The model under review builds one solid part; all positions refer to its coordinate system, in mm. A direction names the side the tool comes from. Coordinates: 2 decimals unless noted, no trailing zeros. Order: outer loops, then holes, each group sorted by start corner. A loop starts at its lowest first (then second) coordinate and runs counter-clockwise, first axis right, second up.
from build123d import *

# Parameters (mm, degrees)
SKETCH_1_W          = 22.9
SKETCH_1_H          = 21
EXTRUDE_1_DEPTH     = 2
SKETCH_2_W          = 4.5
SKETCH_2_H          = 6
EXTRUDE_2_DEPTH     = 14.4
FILLET_1_R          = 1
SKETCH_3_R          = 4
CUT_EXTRUDE_1_DEPTH = 14.4
SKETCH_5_R          = 0.95
CUT_EXTRUDE_2_DEPTH = 14.4
SKETCH_1_2_W        = 22.9
SKETCH_1_2_H        = 21
EXTRUDE_3_DEPTH     = 2
SKETCH_6_R          = 4
CUT_EXTRUDE_3_DEPTH = 1
SKETCH_7_R          = 1.75
CUT_EXTRUDE_4_DEPTH = 1
FILLET_2_R          = 1
SKETCH_9_W          = 22.900603658
SKETCH_9_H          = 0.5
CUT_EXTRUDE_5_DEPTH = 4
FILLET_4_R          = 1
FILLET_5_DEPTH      = 14.4


with BuildPart() as part:
    # 草图1 → 凸台-拉伸1 (new body)
    with BuildSketch(Plane(origin=(0, 0, 0), x_dir=(1, 0, 0), z_dir=(0, 1, 0))):
        Rectangle(SKETCH_1_W, SKETCH_1_H)
    extrude(amount=EXTRUDE_1_DEPTH)

    # 草图2 → 凸台-拉伸2 (add)
    with BuildSketch(Plane(origin=(0, 0, 0), x_dir=(1, 0, 0), z_dir=(0, 1, 0))):
        with Locations((-13.7, -1.1)):
            Rectangle(SKETCH_2_W, SKETCH_2_H)
        with Locations((13.7, -1.1)):
            Rectangle(SKETCH_2_W, SKETCH_2_H)
    extrude(amount=EXTRUDE_2_DEPTH)

    # 圆角1
    fillet_1_edges = [part.edges().sort_by_distance(p)[0] for p in [
        (-11.45, 8.2, 4.1),
        (11.45, 8.2, 4.1),
    ]]
    fillet(fillet_1_edges, radius=FILLET_1_R)

    # 草图3 → 切除-拉伸1 (cut)
    with BuildSketch(Plane(origin=(0, 2, 0), x_dir=(1, 0, 0), z_dir=(0, 1, 0))):
        with Locations(Location((-0.63, -1.66, 0), (0, 0, 270))):
            Circle(SKETCH_3_R)
    extrude(amount=-CUT_EXTRUDE_1_DEPTH, mode=Mode.SUBTRACT)

    # 草图5 → 切除-拉伸2 (cut)
    with BuildSketch(Plane.XY.offset(4.1)):
        with Locations((-13.85, 8.2)):
            Circle(SKETCH_5_R)
        with Locations((13.85, 8.2)):
            Circle(SKETCH_5_R)
    extrude(amount=-CUT_EXTRUDE_2_DEPTH, mode=Mode.SUBTRACT)

    # 草图1<2> → 凸台-拉伸3 (add)
    with BuildSketch(Plane(origin=(0, 0, 0), x_dir=(1, 0, 0), z_dir=(0, 1, 0))):
        Rectangle(SKETCH_1_2_W, SKETCH_1_2_H)
    extrude(amount=-EXTRUDE_3_DEPTH)

    # 草图6 → 切除-拉伸3 (cut)
    with BuildSketch(Plane(origin=(0, 0, 0), x_dir=(1, 0, 0), z_dir=(0, 1, 0))):
        with Locations(Location((-0.63, -1.66, 0), (0, 0, 270))):
            Circle(SKETCH_6_R)
    extrude(amount=-CUT_EXTRUDE_3_DEPTH, mode=Mode.SUBTRACT)

    # 草图7 → 切除-拉伸4 (cut)
    with BuildSketch(Plane(origin=(0, -1, 0), x_dir=(1, 0, 0), z_dir=(0, 1, 0))):
        with Locations(Location((-0.63, -1.66, 0), (0, 0, 270))):
            Circle(SKETCH_7_R)
    extrude(amount=-CUT_EXTRUDE_4_DEPTH, mode=Mode.SUBTRACT)

    # 圆角2
    fillet_2_edges = [part.edges().sort_by_distance(p)[0] for p in [
        (11.45, 0, -10.5),
        (-11.45, 0, -10.5),
    ]]
    fillet(fillet_2_edges, radius=FILLET_2_R)

    # 草图9 → 切除-拉伸5 (cut)
    with BuildSketch(Plane(origin=(0, 2, 0), x_dir=(1, 0, 0), z_dir=(0, 1, 0))):
        with Locations((-0.000301829, -10.25)):
            Rectangle(SKETCH_9_W, SKETCH_9_H)
    extrude(amount=-CUT_EXTRUDE_5_DEPTH, mode=Mode.SUBTRACT)

    # 圆角4
    fillet_4_edges = [part.edges().sort_by_distance(p)[0] for p in [
        (-11.45, 0, 10),
        (11.45, 0, 10),
    ]]
    fillet(fillet_4_edges, radius=FILLET_4_R)

    # 圆角5: read off the stored shape, not the designer's step
    # 圆角5 outline → 圆角5 (cut)
    with BuildSketch(Plane(origin=(0, 0, 0), x_dir=(1, 0, 0), z_dir=(0, 1, 0))):
        with BuildLine():
            ThreePointArc((11.45, 1.9), (14.69341649, -0.235240405), (15.95, -3.909475019))
            Line((15.95, -3.909475019), (15.95, 1.9))
            Line((15.95, 1.9), (11.45, 1.9))
        make_face()
        with BuildLine():
            ThreePointArc((-15.95, -3.909475019), (-14.69341649, -0.235240405), (-11.45, 1.9))
            Line((-11.45, 1.9), (-15.95, 1.9))
            Line((-15.95, 1.9), (-15.95, -3.909475019))
        make_face()
    extrude(amount=FILLET_5_DEPTH, mode=Mode.SUBTRACT)


solid = part.part
(1) Consider section C-C (x = -0.63). Give the boundary of the cut face in (y, z).
(2) Consider section A-A (y = 12.75). Give the boundary of the cut face in (x, z), then the cut area to 3 significant figures.
(3) Wall thickness on line 1 (X direction, y = 8.2, z = 2); line 2 (Y direction, x = -13.85, z = 1.3); line 3 (X direction, y = -0.15, z = 1.66): over which ranges is each line inside the solid? List them lowest first.
(4) Tool access review of faces 1 (the face through (-11.45, 8, 1)), 2 (the face through (13, 0, 2)), 3 (the face through (-1.5, -1, 3.4)), 4 (the face through (14, 7, 4.1)): name each direction out of +Z, -Z, +X, -X, +Y, -Y from which nothing blocks a thin tool from reaching the whole face with its end or side.
(5) The part is to be moulded in two halves that separate along Z. For faces 5 (the face through (0, 2, -3)), 6 (the face through (-0.55, -1.49, -0.09)), 7 (the face through (11.735, 8.287, 3.799)), say which applies: +Z half, -Z half, draft (parallel to the pull), parting line (faces both ways), or undercut.
(6) Consider section D-D (y = 1.5). Give the boundary of the cut face in (x, z).
(7) Consider section B-B (z = 1.66). Give the boundary of the cut face in (x, y), then the cut area to 3 significant figures.
(8) Insertion check: pin 1 Ø3.5 at (x, y) = (12.5, 4) entering from +Z; pin 2 Ø8 at (y, z) = (7.5, 0.5) entering from +X; pin 3 Ø1.5 at (x, y) = (-9.5, 10.5) entering from -Z; pin 4 Ø3.5 at (x, z) = (14.5, 2) entering from -Y. Each pin has a flat end and moves straight along its axis. Give the tip position at first contact, or say it passes through.
Findings:
1. outline: (-2, -10.5) - (2, -10.5) - (2, -2.34) - (-1, -2.34) - (-1, -0.09) - (-2, -0.09) - close; (-2, 3.41) - (-1, 3.41) - (-1, 5.66) - (2, 5.66) - (2, 10) - (-2, 10) - close
2. outline: (-15.95, 3.91) arc R6 ccw to (-11.45, -1.9) - (-11.45, 3.1) arc R1 ccw to (-12.45, 4.1) - (-15.95, 4.1) - close; (11.45, -1.9) arc R6 ccw to (15.95, 3.91) - (15.95, 4.1) - (12.45, 4.1) arc R1 ccw to (11.45, 3.1) - close
2. area: 40.0 mm2
3. line 1: x = -15.64 to -14.8, -12.9 to -11.45, 11.45 to 12.9, 14.8 to 15.64
3. line 2: y = 0 to 7.25, 9.15 to 14.4
3. line 3: x = -11.45 to -4.63, 3.37 to 11.45
4. face 1: +Z, -Z, +Y
4. face 2: +Z, -Z, +X, -Y
4. face 3: +Y
4. face 4: +Z, +X, +Y, -Y
5. face 5: draft
5. face 6: undercut
5. face 7: +Z half
6. outline: (-15.95, 3.91) arc R6 ccw to (-11.45, -1.9) - (-11.45, -9.5) arc R1 ccw to (-10.45, -10.5) - (10.45, -10.5) arc R1 ccw to (11.45, -9.5) - (11.45, -1.9) arc R6 ccw to (15.95, 3.91) - (15.95, 4.1) - (11.45, 4.1) - (11.45, 9) arc R1 ccw to (10.45, 10) - (-10.45, 10) arc R1 ccw to (-11.45, 9) - (-11.45, 4.1) - (-15.95, 4.1) - close; hole circle Ø8 at (-0.63, 1.66)
7. outline: (-15.51, 0) - (-11.45, 0) - (-11.45, -2) - (-2.38, -2) - (-2.38, -1) - (-4.63, -1) - (-4.63, 2) - (-11.45, 2) - (-11.45, 14.4) - (-15.51, 14.4) - close; (1.12, -2) - (11.45, -2) - (11.45, 0) - (15.51, 0) - (15.51, 14.4) - (11.45, 14.4) - (11.45, 2) - (3.37, 2) - (3.37, -1) - (1.12, -1) - close; hole circle Ø1.9 at (-13.85, 8.2); hole circle Ø1.9 at (13.85, 8.2)
7. area: 175 mm2
8. pin 1: stops at z = 4.1
8. pin 2: stops at x = 15.95
8. pin 3: passes through
8. pin 4: stops at y = 0
